Work out the finished part from the listing and answer in its coordinate system (mm). A direction names the side the tool comes from. Give positions to 0.01 mm unless a question says otherwise; leave off trailing zeros. Loops run counter-clockwise (first coordinate to the right, second up) from the corner with the lowest first, then second, coordinate; pieces in that order, holes last. Notation, with made-up numbers: M 17.25,-16 L 37.25,-16 A17 ccw 37.25,-5 Z; hole C 3.5,-9.75 d11. An arc over 180 degrees is marked long. Use a Markdown table: item, result.
Autodesk Inventor part; units mm, degrees
ref_plane "YZ Plane" through (0, 0, 0) normal (1, 0, 0) x (0, 1, 0)
ref_plane "XZ Plane" through (0, 0, 0) normal (0, 1, 0) x (-1, 0, 0)
ref_plane "XY Plane" through (0, 0, 0) normal (0, 0, 1) x (1, 0, 0)
sketch "Sketch1" plane through (0, 0, 0) normal (0, 1, 0) x (-1, 0, 0)
  circle A0 centre (0, 0) radius 45
  circle A1 centre (0, 0) radius 55
  dimension "d0" = 90
  dimension "d1" = 110
extrude "Extrusion1" add sketch "Sketch1" along normal blind 5
sketch "Sketch2" plane through (0, 5, 0) normal (0, 1, 0) x (1, 0, 0)
  circle A0 centre (0, 0) radius 45
  circle A1 centre (0, 0) radius 47
  dimension "d4" = 90
  dimension "d5" = 94
extrude "Extrusion2" cut sketch "Sketch2" against normal blind 2
sketch "Sketch3" plane through (0, 5, 0) normal (0, 1, 0) x (1, 0, 0)
  circle A0 centre (0, -50) radius 1
  circle A1 centre (0, 0) radius 55
  dimension "d8" = 2
  dimension "d9" = 50
hole "Hole1" at (0, 5, 50) direction (0, -1, 0) diameter 2 end through all
sketch "Sketch4" plane through (0, 5, 0) normal (0, 1, 0) x (1, 0, 0)
  circle A0 centre (-50, 0) radius 1
  point P0 (0, 0)
  dimension "d17" = 2
  dimension "d18" = 50
sketch "Sketch5" plane through (0, 5, 0) normal (0, 1, 0) x (1, 0, 0)
  circle A0 centre (0, 50) radius 1
  point P0 (0, 0)
  dimension "d19" = 2
  dimension "d20" = 50
sketch "Sketch6" plane through (0, 5, 0) normal (0, 1, 0) x (1, 0, 0)
  circle A0 centre (50, 0) radius 1
  point P0 (0, 0)
  dimension "d21" = 2
  dimension "d22" = 50
hole "Hole2" at (-50, 5, 0) direction (0, -1, 0) diameter 2 end through all
hole "Hole3" at (0, 5, -50) direction (0, -1, 0) diameter 2 end through all
hole "Hole4" at (50, 5, 0) direction (0, -1, 0) diameter 2 end through all
thread "Thread1"
thread "Thread2"
thread "Thread3"
thread "Thread4"
properties part number "Mirror Support"
(1) Which of the six approach directions +Z, -Z, +X, -X, +Y, -Y give full straight-line access (tool end or side, diameter ignored) to faces 1 (the cylindrical face through (44.83, 4.01, -14.12)), 2 (the flat face through (4, 0, 45))?
Entries:
| item | result |
|---|---|
| face 1 | +Y |
| face 2 | +Z, -Z, +X, -X, -Y |
(2) Consider probe 1 along Z at (x, y) = (0, 1.3); probe 2 along Z at (x, y) = (0, 3.85); probe 3 along X at (y, z) = (1.55, 35). Determine where each line is inside the solid, lowest interval first. Write a range as [from, to].
Entries:
| item | result |
|---|---|
| probe 1 | z = [-55, -51], [-49, -45], [45, 49], [51, 55] |
| probe 2 | z = [-55, -51], [-49, -47], [47, 49], [51, 55] |
| probe 3 | x = [-42.43, -28.28], [28.28, 42.43] |
(3) A cutting plane is placed at B-B (z = -23.5). Write down the section's boundary in (x, y).
Entries:
| item | result |
|---|---|
| outline | M -49.73,0 L -38.38,0 L -38.38,3 L -40.7,3 L -40.7,5 L -49.73,5 Z; M 38.38,0 L 49.73,0 L 49.73,5 L 40.7,5 L 40.7,3 L 38.38,3 Z |
(4) The mould has two halves that part along X. Classify faces 3 (the cylindrical face through (11.923, 2.465, 53.692)), 4 (the flat face through (45.04, 3, 3.26)), 5 (the flat face through (-40.5, 5, -24.2)), 6 (the cylindrical face through (-20.765, 1.479, 39.923)): released by +X, released by -X, zero draft, split by the parting line, or undercut.
Entries:
| item | result |
|---|---|
| face 3 | split by the parting line |
| face 4 | undercut |
| face 5 | zero draft |
| face 6 | undercut |
(5) Given P1, Ø1.5, axis at x = 6, y = 3.5, coming from the -Z side, flat-ended and moving along its own axis, determine where the tip first touches the part or whether it passes through.
Entries:
| item | result |
|---|---|
| P1 | stops at z = -54.75 |
(6) A cutting plane is placed at A-A (x = 30.5). Write down the section's boundary in (y, z).
Entries:
| item | result |
|---|---|
| outline | M 0,-45.77 L 5,-45.77 L 5,-35.76 L 3,-35.76 L 3,-33.09 L 0,-33.09 Z; M 0,33.09 L 3,33.09 L 3,35.76 L 5,35.76 L 5,45.77 L 0,45.77 Z |
(7) A cutting plane is placed at C-C (y = 1.15). Write down the section's boundary in (x, z).
Entries:
| item | result |
|---|---|
| outline | C 0,0 d110; hole C -50,0 d2; hole C 0,0 d90; hole C 0,-50 d2; hole C 0,50 d2; hole C 50,0 d2 |
